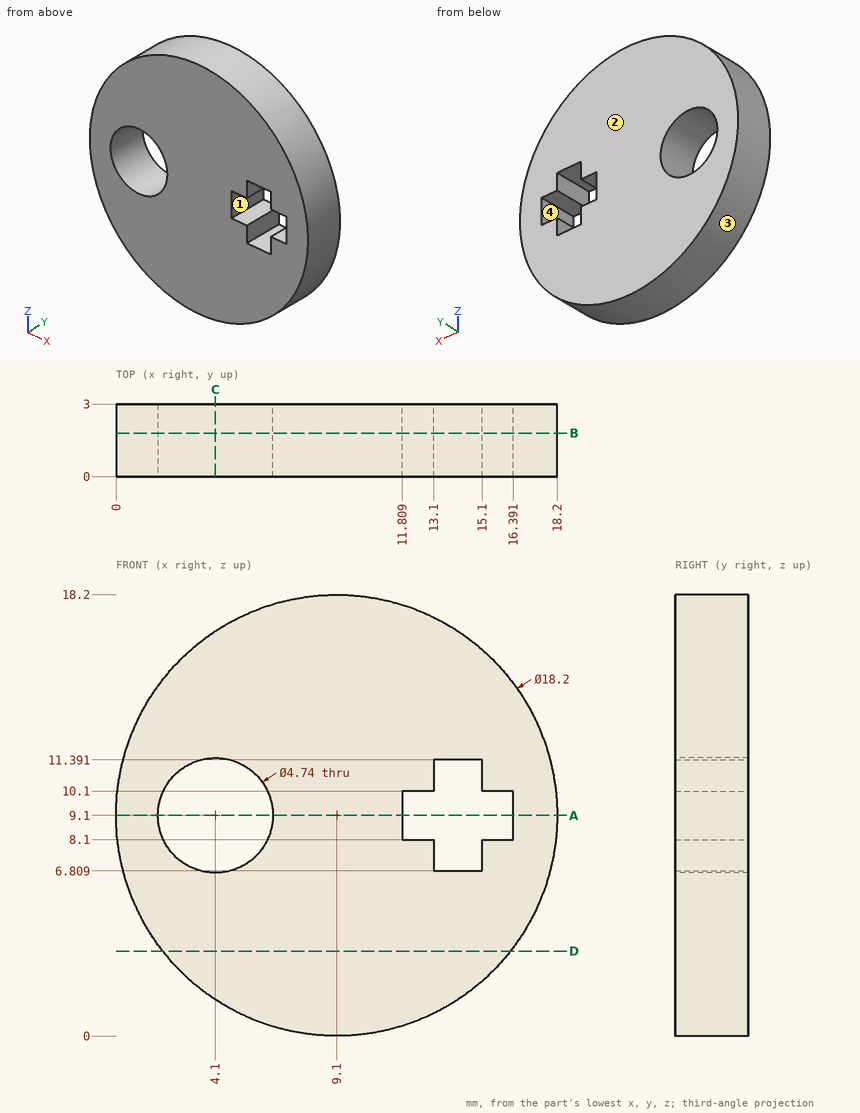
Here's the drawing with two shaded views (mm, measured from the low corner). I have some questions. Give positions to 0.01 mm unless a question says otherwise; leave off trailing zeros. Loops run counter-clockwise (first coordinate to the right, second up) from the corner with the lowest first, then second, coordinate; pieces in that order, holes last. Notation, with made-up numbers: M 57.5,84.5 L 94.5,84.5 A13 cw 94.5,91.5 Z; hole C 25.25,-15 d4. An arc over 180 degrees is marked long. Use one line per item in the form item = value. Start each with the question number.
Q1. If we section it at D-D (z = 3.5): Write out the boundary of the cut face in (x, y).
Q2. I need wall thicknesses on line 1 along X through (y, z) = (1.25, 9); line 2 along X through (y, z) = (2.3, 10.75); line 3 along Z through (x, y) = (3.75, 2.6) (1 decimal). Which ranges of each line are inside material? Lowest first, please.
Q3. Thinking about a two-plate mould opening in X: for the marked faces 1, 2, 3 and 4, which applies, +X half, -X half, draft (parallel to the pull), parting line (faces both ways), or undercut?
Q4. If we section it at A-A (z = 9.1): Write out the boundary of the cut face in (x, y).
Q5. If we section it at C-C (x = 4.1): Write out the boundary of the cut face in (y, z).
Q6. Will these pins go through, and if not, where does the flat tip stop? pin 1 Ø1.4 at (y, z) = (1.5, 10.5) entering from +X; pin 2 Ø8 at (x, z) = (16, 8.5) entering from +Y; pin 3 Ø0.6 at (x, y) = (15.5, 2) entering from +Z; pin 4 Ø1.6 at (x, y) = (13.5, 2) entering from -Z.
Q7. If we section it at B-B (y = 1.8): Write out the boundary of the cut face in (x, z).
Taken from the geometry:
q1.outline = M 1.93,0 L 16.27,0 L 16.27,3 L 1.93,3 Z
q2.line_1 = 0 to 1.73, 6.47 to 11.81, 16.39 to 18.2
q2.line_2 = 0.15 to 2.4, 5.8 to 13.1, 15.1 to 18.05
q2.line_3 = 1.7 to 6.8, 11.4 to 16.5
q3.face_1 = undercut
q3.face_2 = draft
q3.face_3 = parting line
q3.face_4 = undercut
q4.outline = M 0,0 L 1.73,0 L 1.73,3 L 0,3 Z; M 6.47,0 L 11.81,0 L 11.81,3 L 6.47,3 Z; M 16.39,0 L 18.2,0 L 18.2,3 L 16.39,3 Z
q5.outline = M 0,1.5 L 3,1.5 L 3,6.73 L 0,6.73 Z; M 0,11.47 L 3,11.47 L 3,16.7 L 0,16.7 Z
q6.pin_1 = 18.17
q6.pin_2 = 3
q6.pin_3 = 15.85
q6.pin_4 = 0.74
q7.outline = C 9.1,9.1 d18.2; hole C 4.1,9.1 d4.74; hole M 11.81,8.1 L 13.1,8.1 L 13.1,6.81 L 15.1,6.81 L 15.1,8.1 L 16.39,8.1 L 16.39,10.1 L 15.1,10.1 L 15.1,11.39 L 13.1,11.39 L 13.1,10.1 L 11.81,10.1 Z
